Geometry check sheet. Reference: the model listing, model coordinates, mm. Face numbers are marked on the shaded views. Round coordinates to 2 decimals unless told otherwise and drop trailing zeros. Write each loop counter-clockwise with the first axis right and the second up, starting at its lowest first coordinate (ties: lowest second). Pieces come first, ordered by that corner, then holes. Notation, with made-up numbers: M 15,89 L 28,89 A13 cw 28,93 Z; hole C -24,88 d9. An arc over 180 degrees is marked long. Answer in a Markdown table with one row per item. Add a question column.
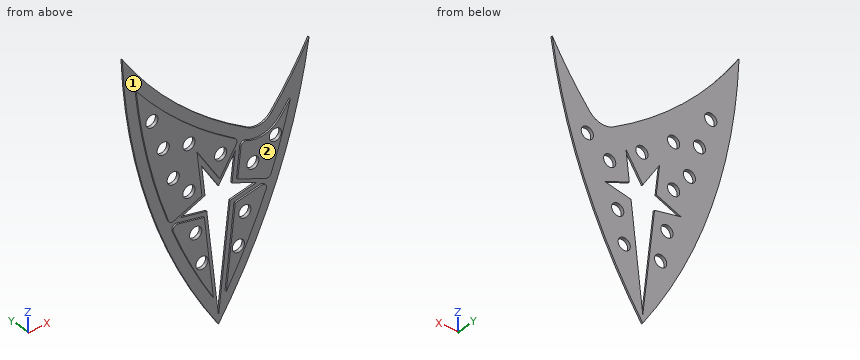
from build123d import *

# Parameters (mm, degrees)
SKETCH4_R             = 1.5
BOSS_EXTRUDE1_DEPTH   = 0.4
BOSS_EXTRUDE1_2_DEPTH = 0.4
BOSS_EXTRUDE1_3_DEPTH = 0.4
BOSS_EXTRUDE1_4_DEPTH = 0.4
SKETCH5_R             = 1.5
BOSS_EXTRUDE2_DEPTH   = 0.4


with BuildPart() as part:
    # Sketch4 → Boss-Extrude1 (new body)
    with BuildSketch(Plane(origin=(0, 0, 0), x_dir=(1, 0, 0), z_dir=(0, 1, 0))):
        with BuildLine():
            Line((36.631982775, 48.402124759), (29.724109313, 45.552485279))
            Line((29.724109313, 45.552485279), (30.536926129, 38.325609907))
            ThreePointArc((30.536926129, 38.325609907), (31.037916291, 37.567202472), (31.94599849, 37.527709405))
            ThreePointArc((31.94599849, 37.527709405), (36.434517541, 37.979126286), (40.266354995, 35.59845365))
            ThreePointArc((40.266354995, 35.59845365), (41.495664758, 34.067994846), (42.693859526, 32.513055637))
            ThreePointArc((42.693859526, 32.513055637), (40.547573161, 40.24119879), (37.949447695, 47.829379455))
            ThreePointArc((37.949447695, 47.829379455), (37.412017647, 48.394779577), (36.631982775, 48.402124759))
        make_face()
        with Locations((33.472, 43.307)):
            Circle(SKETCH4_R, mode=Mode.SUBTRACT)
        with Locations((38.989, 39.243)):
            Circle(SKETCH4_R, mode=Mode.SUBTRACT)
    extrude(amount=BOSS_EXTRUDE1_DEPTH)



with BuildPart() as body_2:
    # Sketch4 → Boss-Extrude1 2 (new body)
    with BuildSketch(Plane(origin=(0, 0, 0), x_dir=(1, 0, 0), z_dir=(0, 1, 0))):
        with BuildLine():
            Line((26.913796721, 70.539393135), (29.126057014, 50.869857351))
            Line((29.126057014, 50.869857351), (35.62874213, 49.537078309))
            ThreePointArc((35.62874213, 49.537078309), (36.597764867, 49.876549859), (36.756875392, 50.890911647))
            ThreePointArc((36.756875392, 50.890911647), (32.232858108, 60.91429454), (26.913796721, 70.539393135))
        make_face()
        with Locations((31.496, 53.848)):
            Circle(SKETCH4_R, mode=Mode.SUBTRACT)
        with Locations((29.901, 61.2)):
            Circle(SKETCH4_R, mode=Mode.SUBTRACT)
    extrude(amount=BOSS_EXTRUDE1_2_DEPTH)


with BuildPart() as body_3:
    # Sketch4 → Boss-Extrude1 3 (new body)
    with BuildSketch(Plane(origin=(0, 0, 0), x_dir=(1, 0, 0), z_dir=(0, 1, 0))):
        with BuildLine():
            Line((20.913318286, 45.552485279), (14.005444824, 48.402124759))
            ThreePointArc((14.005444824, 48.402124759), (13.225409952, 48.394779577), (12.687979904, 47.829379455))
            ThreePointArc((12.687979904, 47.829379455), (7.625203146, 31.191555875), (4.727035456, 14.043684112))
            ThreePointArc((4.727035456, 14.043684112), (15.974402208, 25.962258497), (29.061917895, 35.824946131))
            ThreePointArc((29.061917895, 35.824946131), (29.505500168, 36.453855806), (29.370974364, 37.211612641))
            Line((29.370974364, 37.211612641), (25.3187138, 43.52403979))
            Line((25.3187138, 43.52403979), (19.700923362, 34.77290143))
            Line((19.700923362, 34.77290143), (20.913318286, 45.552485279))
        make_face()
        with Locations((8.58, 22.733)):
            Circle(SKETCH4_R, mode=Mode.SUBTRACT)
        with Locations((11.374, 30.353)):
            Circle(SKETCH4_R, mode=Mode.SUBTRACT)
        with Locations((13.843, 38.354)):
            Circle(SKETCH4_R, mode=Mode.SUBTRACT)
        with Locations((17.724, 32.004)):
            Circle(SKETCH4_R, mode=Mode.SUBTRACT)
        with Locations((17.724, 43.18)):
            Circle(SKETCH4_R, mode=Mode.SUBTRACT)
        with Locations((25.527, 37.846)):
            Circle(SKETCH4_R, mode=Mode.SUBTRACT)
    extrude(amount=BOSS_EXTRUDE1_3_DEPTH)


with BuildPart() as body_4:
    # Sketch4 → Boss-Extrude1 4 (new body)
    with BuildSketch(Plane(origin=(0, 0, 0), x_dir=(1, 0, 0), z_dir=(0, 1, 0))):
        with BuildLine():
            Line((15.008685469, 49.537078309), (21.511370585, 50.869857351))
            Line((21.511370585, 50.869857351), (23.723630878, 70.539393135))
            ThreePointArc((23.723630878, 70.539393135), (18.404569491, 60.91429454), (13.880552207, 50.890911647))
            ThreePointArc((13.880552207, 50.890911647), (14.039662732, 49.876549859), (15.008685469, 49.537078309))
        make_face()
        with Locations((19.375, 53.594)):
            Circle(SKETCH4_R, mode=Mode.SUBTRACT)
        with Locations((20.925, 61.225)):
            Circle(SKETCH4_R, mode=Mode.SUBTRACT)
    extrude(amount=BOSS_EXTRUDE1_4_DEPTH)


with BuildPart() as part_1:
    add(part.part)

    add(body_2.part)  # Boss-Extrude2 merges body 2

    add(body_3.part)  # Boss-Extrude2 merges body 3

    add(body_4.part)  # Boss-Extrude2 merges body 4
    # Sketch5 → Boss-Extrude2 (add)
    with BuildSketch(Plane(origin=(0, 0.4, 0), x_dir=(1, 0, 0), z_dir=(0, 1, 0))):
        with BuildLine():
            ThreePointArc((25.3187138, 77.655988793), (8.417285199, 43.223132296), (1.60825988, 5.475058578))
            ThreePointArc((1.60825988, 5.475058578), (15.395050063, 22.022293224), (32.560079542, 35.031840527))
            ThreePointArc((32.560079542, 35.031840527), (35.635218263, 35.591596594), (38.333143822, 34.01330553))
            ThreePointArc((38.333143822, 34.01330553), (43.27239761, 27.425793547), (47.621637666, 20.434681115))
            ThreePointArc((47.621637666, 20.434681115), (39.681799875, 50.297117055), (25.3187138, 77.655988793))
        make_face()
        with Locations((8.58, 22.733)):
            Circle(SKETCH5_R, mode=Mode.SUBTRACT)
        with Locations((11.374, 30.353)):
            Circle(SKETCH5_R, mode=Mode.SUBTRACT)
        with Locations((17.724, 43.18)):
            Circle(SKETCH5_R, mode=Mode.SUBTRACT)
        with Locations((13.843, 38.354)):
            Circle(SKETCH5_R, mode=Mode.SUBTRACT)
        with Locations((17.724, 32.004)):
            Circle(SKETCH5_R, mode=Mode.SUBTRACT)
        with Locations((38.989, 39.243)):
            Circle(SKETCH5_R, mode=Mode.SUBTRACT)
        with Locations((33.472, 43.307)):
            Circle(SKETCH5_R, mode=Mode.SUBTRACT)
        with Locations((31.496, 53.848)):
            Circle(SKETCH5_R, mode=Mode.SUBTRACT)
        with Locations((29.901, 61.2)):
            Circle(SKETCH5_R, mode=Mode.SUBTRACT)
        with Locations((20.925, 61.225)):
            Circle(SKETCH5_R, mode=Mode.SUBTRACT)
        with Locations((19.375, 53.594)):
            Circle(SKETCH5_R, mode=Mode.SUBTRACT)
        with Locations((25.527, 37.846)):
            Circle(SKETCH5_R, mode=Mode.SUBTRACT)
        Polygon((22.423901789, 50.036100284), (25.3187138, 75.774305051), (28.21352581, 50.036100284), (34.731994844, 48.700086198), (28.646152557, 46.189551437), (29.464018945, 38.917779558), (25.3187138, 45.375147323), (21.173408654, 38.917779558), (21.991275042, 46.189551437), (15.905432755, 48.700086198), align=None, mode=Mode.SUBTRACT)
    extrude(amount=BOSS_EXTRUDE2_DEPTH)


solid = part_1.part
Item 1: Section check C-C, the plane z = -57. Record the boundary of the cut face in (x, y), and give its area (3 significant figures).
Item 2: Mould release check, pull along Z, two halves, no side actions. Record for the marked faces 1 and 2: +Z half, -Z half, draft (parallel to the pull), parting line (faces both ways), or undercut.
Item 3: Scan lines: probe 1 along Z at (x, y) = (19, 0.05); probe 2 along Z at (x, y) = (34, 0.1); probe 3 along X at (y, z) = (0.5, -61.2). Record each from-to range of solid material in increasing order. Write a range as from..to.
Item 4: Gauge pin test, flat end, axial feed: pin 1 Ø2.5 at (x, z) = (31.496, -53.848) entering from -Y. Record the tip position at first contact, or that the pin passes through.
Item 5: Section check B-B, the plane y = 0.65. Give the number of separate pieces and of enclosed holes in the cut face, and give its area (3 significant figures).
Item 6: Section check A-A, the plane x = 8.58. Record the boundary of the cut face in (y, z), and give its area (3 significant figures).
Result sheet:
| question | item | result |
|---|---|---|
| 1 | outline | M 13.77,0.4 L 16.52,0.4 L 16.52,0 L 22.2,0 L 22.2,0.4 L 23.21,0.4 L 23.21,0.8 L 13.77,0.8 Z; M 27.43,0.4 L 28.44,0.4 L 28.44,0 L 34.12,0 L 34.12,0.4 L 36.86,0.4 L 36.86,0.8 L 27.43,0.8 Z |
| 1 | area | 12.1 mm^2 |
| 2 | face 1 | undercut |
| 2 | face 2 | draft |
| 3 | probe 1 | z = -62.09..-55.05, -52.14..-50.36, -46.34..-43.97, -42.39..-32.79, -31.22..-28.56 |
| 3 | probe 2 | z = -57.25..-49.87, -47.32..-44.71, -41.9..-38.11 |
| 3 | probe 3 | x = 15.76..19.43, 22.42..23.68, 26.96..28.4, 31.4..34.88 |
| 4 | pin 1 | passes through |
| 5 | separate pieces | 1 |
| 5 | enclosed holes | 13 |
| 5 | area | 1,100 mm^2 |
| 6 | outline | M 0,-35 L 0.4,-35 L 0.4,-43.72 L 0.8,-43.72 L 0.8,-24.23 L 0,-24.23 Z; M 0,-21.23 L 0.8,-21.23 L 0.8,-14.8 L 0.4,-14.8 L 0.4,-18.59 L 0,-18.59 Z |
| 6 | area | 15.7 mm^2 |
